CAD build for the part. Positions are in the model's coordinates, mm. A direction names the side the tool comes from. Coordinates: 2 decimals unless noted, no trailing zeros. Order: outer loops, then holes, each group sorted by start corner. A loop starts at its lowest first (then second) coordinate and runs counter-clockwise, first axis right, second up. Notation, with made-up numbers: M -16,-37 L -6,-37 A7 cw -6,-32 Z; hole C 69.25,-4.75 d4. An arc over 180 degrees is marked long. One line per item, written item: value.
from build123d import *

# Parameters (mm, degrees)
F0_W = 2.4999999441
F0_H = 10.1996297166


# Not quite as in the source:
# - ends of sketch curves that miss each other by under 0.0002 mm in the source are joined


with BuildPart() as f1:
    # F0 (on Front) → F1 (revolve)
    with BuildSketch(Plane.XZ):
        Polygon((0, -34.0000009239), (0, -10.1996297166), (-2.4999999441, -10.1996297166), (-6.5000001341, -10.1996297166), (-6.5000001341, -34), (-0.75, -34), align=None)
        with Locations((-1.2499999721, -5.0998148583)):
            Rectangle(F0_W, F0_H)
        Polygon((0, 2.3), (-10, 2.3), (-10, 0), (-2.4999999441, 0), (0, 0), align=None)
        Polygon((0, -40.7000018477), (0, -34.0000009239), (-0.75, -34), (-0.75, -40.7000018477), align=None)
    revolve(axis=Axis((0, 0, -22.5782128982), (0, 0, -1)))


solid = f1.part
Q1. Slice it at B-B (x = 0). List the corners of the cut face in (y, z).
Recorded:
outline: M -10,0 L -2.5,0 L -2.5,-10.2 L -6.5,-10.2 L -6.5,-34 L -0.75,-34 L -0.75,-40.7 L 0.75,-40.7 L 0.75,-34 L 6.5,-34 L 6.5,-10.2 L 2.5,-10.2 L 2.5,0 L 10,0 L 10,2.3 L -10,2.3 Z
Q2. Which spindle directions (+Z, -Z, +X, -X, +Y, -Y) get a long thin tool onto all of the face, cutting with end or side? Do faces 1 (the face through (0.75, 0.03, -37.4)), 2 (the face through (0, 0, -40.7)), 3 (the face through (3, 0, -10.2)). Say none if no direction does.
Recorded:
face 1: -Z
face 2: -Z, +X, -X, +Y, -Y
face 3: none
Q3. Drill centre lines: line 1 along Z through (x, y) = (-3.5, 0.25); line 2 along Z through (x, y) = (7, -1.75); line 3 along X through (y, z) = (7, 0.5). Where is each one in solid material? Low to high.
Recorded:
line 1: z = -34 to -10.2, 0 to 2.3
line 2: z = 0 to 2.3
line 3: x = -7.14 to 7.14
Q4. Pin check, flat tips, straight feed: pin 1 Ø6 at (x, z) = (-7.5, -8) entering from -Y; pin 2 Ø10 at (x, z) = (2.5, -25.5) entering from +Y; pin 3 Ø4 at (y, z) = (-4, -10.5) entering from +X; pin 4 Ø10.5 at (x, y) = (-1.5, 0) entering from -Z. Stop position of each tip, or through.
Recorded:
pin 1: stops at y = -3.53
pin 2: stops at y = 6.5
pin 3: stops at x = 6.18
pin 4: stops at z = -40.7
Q5. Slice it at A-A (x = -3.5). List the corners of the cut face in (y, z), plus the area to 3 significant figures.
Recorded:
outline: M -9.37,0 L 9.37,0 L 9.37,2.3 L -9.37,2.3 Z; M -5.48,-34 L 5.48,-34 L 5.48,-10.2 L -5.48,-10.2 Z
area: 304 mm^2
Q6. Slice it at C-C (y = 4.5). List the corners of the cut face in (x, z), plus the area to 3 significant figures.
Recorded:
outline: M -8.93,0 L 8.93,0 L 8.93,2.3 L -8.93,2.3 Z; M -4.69,-34 L 4.69,-34 L 4.69,-10.2 L -4.69,-10.2 Z
area: 264 mm^2
